Input: part model. Units: mm. Frame: model coordinates. Coordinates: 2 decimals unless noted, no trailing zeros. Order: outer loops, then holes, each group sorted by start corner. A loop starts at its lowest first (then second) coordinate and runs counter-clockwise, first axis right, second up. Notation, with made-up numbers: M -3.75,20 L 8.25,20 A23 ccw 8.25,32 Z; hole C -27.5,48.5 d3. An arc over 180 degrees is marked long. Answer in a Markdown table with one row per item.
from build123d import *

# Parameters (mm, degrees)
F0_W     = 125
F0_H     = 15
F0_R     = 2.5
F0_R_2   = 3.25
F1_DEPTH = 12
F2_SIZE  = 2.75
F3_SIZE  = 0.5


with BuildPart() as f1:
    # F0 (on Front) → F1 (new body)
    with BuildSketch(Plane.XZ):
        with Locations((-21.2495, 0)):
            Rectangle(F0_W, F0_H)
        with Locations((-76.7495, 0)):
            Circle(F0_R, mode=Mode.SUBTRACT)
        with Locations((-63.7495, 0)):
            Circle(F0_R, mode=Mode.SUBTRACT)
        with Locations((-50.7495, 0)):
            Circle(F0_R, mode=Mode.SUBTRACT)
        with Locations((-21.2495, 0)):
            Circle(F0_R_2, mode=Mode.SUBTRACT)
        with Locations((3.7505, 0)):
            Circle(F0_R_2, mode=Mode.SUBTRACT)
        with Locations((28.7505, 0)):
            Circle(F0_R_2, mode=Mode.SUBTRACT)
    extrude(amount=F1_DEPTH)

    # F2
    f2_edges = [f1.edges().sort_by_distance(p)[0] for p in [
        (-24.4995, -12, 0),
        (0.5005, -12, 0),
        (25.5005, -12, 0),
    ]]
    chamfer(f2_edges, length=F2_SIZE)

    # F3
    f3_edges = [f1.edges().sort_by_distance(p)[0] for p in [
        (-79.2495, -12, 0),
        (-66.2495, -12, 0),
        (-53.2495, -12, 0),
        (0.5005, 0, 0),
        (25.5005, 0, 0),
        (-24.4995, 0, 0),
        (-53.2495, 0, 0),
        (-66.2495, 0, 0),
        (-79.2495, 0, 0),
    ]]
    chamfer(f3_edges, length=F3_SIZE)


solid = f1.part
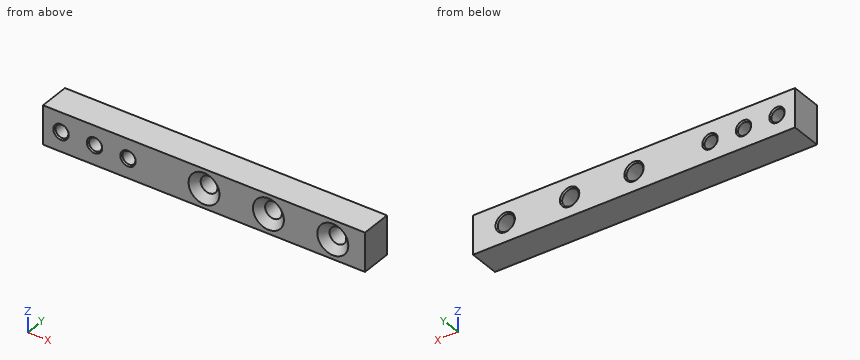
1) Cut plane B-B, the plane z = 0. State how many separate pieces and enclosed holes the cut face has, and give its area (3 significant figures).
Resolved:
| item | result |
|---|---|
| separate pieces | 7 |
| enclosed holes | 0 |
| area | 1,060 mm2 |
2) Cut plane A-A, the plane y = -7. Output: boundary loops of the cut face in (x, z), and give its area (3 significant figures).
Resolved:
| item | result |
|---|---|
| outline | M -83.75,-7.5 L 41.25,-7.5 L 41.25,7.5 L -83.75,7.5 Z; hole C -76.75,0 d5; hole C -63.75,0 d5; hole C -50.75,0 d5; hole C -21.25,0 d6.5; hole C 3.75,0 d6.5; hole C 28.75,0 d6.5 |
| area | 1,720 mm2 |
3) Contact query for a flat-ended pin moving along its axis: pin 1 (8.5 mm diameter, centred on x = 28.75, z = 0, fed in from -Y). Output: stop coordinate, or through.
Resolved:
| item | result |
|---|---|
| pin 1 | stops at y = -10.25 |
4) Material intervals for probe 1 along Z at (x, y) = (-63.5, -7.5); probe 2 along Z at (x, y) = (29, -5.5); probe 3 along X at (y, z) = (-5.5, -3), sorted ascending.
Resolved:
| item | result |
|---|---|
| probe 1 | z = -7.5 to -2.49, 2.49 to 7.5 |
| probe 2 | z = -7.5 to -3.24, 3.24 to 7.5 |
| probe 3 | x = -83.75 to -22.5, -20 to 2.5, 5 to 27.5, 30 to 41.25 |
